```python
from build123d import *

# Parameters (mm, degrees)
F0_W     = 9.81
F0_H     = 2
F1_DEPTH = 15.75
F2_R     = 5
F3_R     = 7
F3_R_2   = 5
F4_DEPTH = 15.3
F5_R     = 7
F5_R_2   = 5
F6_DEPTH = 15.3
F8_DEPTH = 15.75


with BuildPart() as f1:
    # F0 (on Front) → F1 (new body)
    with BuildSketch(Plane.XZ):
        Polygon((-9.81, 22.150199), (-11.81, 22.150199), (-11.81, -6.849801), (-9.81, -6.849801), (-9.81, -4.849801), align=None)
        with Locations((-4.905, -5.849801)):
            Rectangle(F0_W, F0_H)
        with Locations((4.905, -5.849801)):
            Rectangle(F0_W, F0_H)
        Polygon((9.81, 22.150199), (9.81, -4.849801), (9.81, -6.849801), (11.81, -6.849801), (11.81, 22.150199), align=None)
    extrude(amount=F1_DEPTH)

    # F2
    f2_edges = [f1.edges().sort_by_distance(p)[0] for p in [
        (10.81, -15.75, 22.150199),
        (-10.81, -15.75, 22.150199),
        (10.81, 0, 22.150199),
        (-10.81, 0, 22.150199),
    ]]
    fillet(f2_edges, radius=F2_R)

    # F3 (on face) → F4 (join)
    with BuildSketch(Plane.YZ.offset(11.81)):
        with Locations((-7.951076, 1.150199)):
            Circle(F3_R)
        with Locations((-7.951076, 1.150199)):
            Circle(F3_R_2, mode=Mode.SUBTRACT)
    extrude(amount=F4_DEPTH)

    # F5 (on face) → F6 (join)
    with BuildSketch(Plane(origin=(0, 0, -6.849801), x_dir=(1, 0, 0), z_dir=(0, 0, -1))):
        with Locations((0, 7.875)):
            Circle(F5_R)
        with Locations((0, 7.875)):
            Circle(F5_R_2, mode=Mode.SUBTRACT)
    extrude(amount=F6_DEPTH)

    # F7 (on face) → F8 (join, through all)
    with BuildSketch(Plane.XZ.offset(15.75)):
        with BuildLine():
            ThreePointArc((9.81, 4.885641), (9.810285, 4.960485), (9.81, 5.035329))
            Line((9.81, 5.035329), (9.81, 4.885641))
        make_face()
        with BuildLine():
            ThreePointArc((-9.81, 5.035329), (-9.810285, 4.960485), (-9.81, 4.885641))
            Line((-9.81, 4.885641), (-9.81, 5.035329))
        make_face()
        with BuildLine():
            Line((-9.81, -4.849801), (0, -4.849801))
            ThreePointArc((0, -4.849801), (-6.910407, -2.002845), (-9.81, 4.885641))
            Line((-9.81, 4.885641), (-9.81, -4.849801))
        make_face()
        with BuildLine():
            Line((9.81, -4.849801), (9.81, 4.885641))
            ThreePointArc((9.81, 4.885641), (6.910407, -2.002846), (0, -4.849801))
            Line((0, -4.849801), (9.81, -4.849801))
        make_face()
    extrude(amount=-F8_DEPTH)


solid = f1.part
```
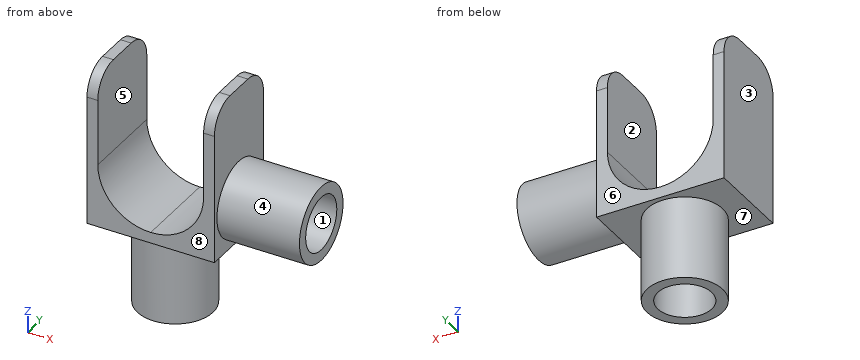
Check sheet for the modelled part. Datum: model origin and axes. Units: mm. Face numbers are marked on the shaded views. A direction names the side the tool comes from. Coordinates: 2 decimals unless noted, no trailing zeros. Order: outer loops, then holes, each group sorted by start corner. A loop starts at its lowest first (then second) coordinate and runs counter-clockwise, first axis right, second up. Notation, with made-up numbers: M 20,-27.5 L 60,-27.5 A32 ccw 60,5.5 Z; hole C 71,-12 d2. An arc over 180 degrees is marked long. One line per question, with ' | ' between items. Start each with the question number.
Item 1: Sectioned sample at A-A on z = 16. Record the cut outline in (x, y), and give its area (3 significant figures).
Item 2: Sectioned sample at D-D on x = 14. Record the cut outline in (y, z).
Item 3: Material ranges on line 1 (Y direction, x = 0, z = -18) (3 decimals); line 2 (X direction, y = -5, z = 14); line 3 (Z direction, x = 24.5, y = -8), recorded low to high.
Item 4: Sectioned sample at C-C on y = -12.25. Record the cut outline in (x, z), and give its area (3 significant figures).
Item 5: Mould release check, pull along X, two halves, no side actions. Record for the marked faces 1, 2 and 3: pulls with the +X half, pulls with the -X half, needs draft (parallel to the pull), parting line crosses it, or undercut.
Item 6: Access from +Z, -Z, +X, -X, +Y, -Y to the whole of each face (thin tool, end or side, straight path). Record for the marked faces 4, 5, 6, 7 and 8.
Item 7: Sectioned sample at B-B on x = 2.5. Record the cut outline in (y, z).
Item 8: Gauge pin test, flat ends, axial feed: P1, Ø8, axis at x = 4.5, z = -3.5, coming from the +Y side; P2, Ø8, axis at x = 0, y = -7.875, coming from the -Z side; P3, Ø2, axis at x = 12, y = -3, coming from the +Z side; P4, Ø4.5, axis at y = -4.5, z = 15, coming from the +X side. Record the tip position at first contact, or that the pin passes through.
Answer below:
1) outline: M -11.81,-15.75 L -9.81,-15.75 L -9.81,0 L -11.81,0 Z; M 9.81,-15.75 L 11.81,-15.75 L 11.81,0 L 9.81,0 Z | area: 63.0 mm^2
2) outline: C -7.95,1.15 d14; hole C -7.95,1.15 d10
3) line 1: y = -14.875 to -12.875, -2.875 to -0.875 | line 2: x = -11.81 to -9.81, 9.81 to 11.81 | line 3: z = -5.85 to -3.85, 6.15 to 8.15
4) outline: M -11.81,-6.85 L -5.46,-6.85 L -5.46,-22.15 L -2.42,-22.15 L -2.42,-6.85 L 2.42,-6.85 L 2.42,-22.15 L 5.46,-22.15 L 5.46,-6.85 L 11.81,-6.85 L 11.81,-4.37 L 27.11,-4.37 L 27.11,-1.4 L 11.81,-1.4 L 11.81,3.7 L 27.11,3.7 L 27.11,6.67 L 11.81,6.67 L 11.81,21.92 L 9.81,21.92 L 9.81,4.89 A9.81 cw 0,-4.85 A9.81 cw -9.81,4.89 L -9.81,21.92 L -11.81,21.92 Z | area: 380 mm^2
5) face 1: needs draft | face 2: undercut | face 3: pulls with the -X half
6) face 4: +X | face 5: +Z, +Y, -Y | face 6: +Z, -Z, +X, -X, +Y | face 7: -Z | face 8: +Z, -Z, +X, -X, -Y
7) outline: M -15.75,-6.85 L -14.41,-6.85 L -14.41,-22.15 L -12.21,-22.15 L -12.21,-6.85 L -3.54,-6.85 L -3.54,-22.15 L -1.34,-22.15 L -1.34,-6.85 L 0,-6.85 L 0,-4.53 L -15.75,-4.53 Z
8) P1: stops at y = 0 | P2: stops at z = -6.85 | P3: stops at z = 22.05 | P4: stops at x = 11.81
